```python
from build123d import *

# Parameters (mm, degrees)
F0_W     = 63.5
F0_H     = 15.24
F1_DEPTH = 4.826
F2_W     = 2.667
F2_H     = 5.715
F2_W_2   = 5.715
F2_H_2   = 1.905
F3_DEPTH = 3.175
F4_W     = 63.5
F4_H     = 15.24
F5_DEPTH = 2.54
F7_D     = 7.1374
F8_R     = 5.08


with BuildPart() as f1:
    # F0 (on Top) → F1 (new body)
    with BuildSketch(Plane.XY):
        Rectangle(F0_W, F0_H)
        Polygon((-3.2995567884, -5.715), (-6.5991135768, 0), (-3.2995567884, 5.715), (3.2995567884, 5.715), (6.5991135768, 0), (3.2995567884, -5.715), align=None, mode=Mode.SUBTRACT)
    extrude(amount=F1_DEPTH)

    # F2 (on face) → F3 (join)
    with BuildSketch(Plane.XY.offset(4.826)):
        with Locations((-30.4165, 0)):
            Rectangle(F2_W, F2_H)
        with Locations((-18.1081227605, -6.6675)):
            Rectangle(F2_W_2, F2_H_2)
        with Locations((18.1081227605, -6.6675)):
            Rectangle(F2_W_2, F2_H_2)
        with Locations((-18.1081227605, 6.6675)):
            Rectangle(F2_W_2, F2_H_2)
        with Locations((18.1081227605, 6.6675)):
            Rectangle(F2_W_2, F2_H_2)
        with Locations((30.4165, 0)):
            Rectangle(F2_W, F2_H)
    extrude(amount=F3_DEPTH)

    # F4 (on face) → F5 (join)
    with BuildSketch(Plane(origin=(0, 0, 0), x_dir=(1, 0, 0), z_dir=(0, 0, -1))):
        Rectangle(F4_W, F4_H)
    extrude(amount=F5_DEPTH)

    # F7 (through all)
    with Locations(Plane(origin=(0, 0, -2.54), x_dir=(1, 0, 0), z_dir=(0, 0, -1))):
        with Locations((0, 0)):
            Hole(F7_D / 2)

    # F8
    f8_edges = [f1.edges().sort_by_distance(p)[0] for p in [
        (31.75, -7.62, 1.143),
        (31.75, 7.62, 1.143),
        (-31.75, 7.62, 1.143),
        (-31.75, -7.62, 1.143),
    ]]
    fillet(f8_edges, radius=F8_R)


solid = f1.part
```
The listing builds one solid part. Answer for the finished solid, in the listing's coordinates (mm). A direction names the side the tool comes from. Round coordinates to 2 decimals unless told otherwise and drop trailing zeros. Write each loop counter-clockwise with the first axis right and the second up, starting at its lowest first coordinate (ties: lowest second). Pieces come first, ordered by that corner, then holes. Notation, with made-up numbers: (63, 68.25) -> (67, 68.25) arc R21 cw to (67, 101.25) -> close; hole circle Ø8 at (86, 4.25). An arc over 180 degrees is marked (long way). Answer as a JSON object with one key per item and string values. Group by question number.
Q1. Section C-C (x = 16) is taken. Write down the section's boundary in (y, z) (3 decimals), plus the area to 3 significant figures.
Q2. Straight lines are drawn through the part: line 1 along Y through (x, z) = (0, -1.1); line 2 along Y through (x, z) = (-1.5, 3.5) (3 decimals); line 3 along X through (y, z) = (6, 5). For each, find the intervals that lie inside material, in ascending order.
Q3. Section D-D (x = -23) is taken. Write down the section's boundary in (y, z).
Q4. Section B-B (x = 0) is taken. Write down the section's boundary in (y, z) (3 decimals).
Q5. Section A-A (z = 1) is taken. Write down the section's boundary in (x, y) (3 decimals).
Q6. Determine the mould class of faces 4 (the face through (-4.97, 2.82, 2.38)), 5 (the face through (30.222, -6.171, 1.633)), 6 (the face through (30, -2.858, 6)) for opening direction X: pulls with the +X half, pulls with the -X half, needs draft (parallel to the pull), parting line crosses it, or undercut.
Q7. Which of the six approach directions +Z, -Z, +X, -X, +Y, -Y give full straight-line access (tool end or side, diameter ignored) to faces 1 (the face through (15.251, 7, 6)), 2 (the face through (-30, -2.858, 6)), 3 (the face through (18, 5.715, 6))?
Q8. Each of these flat-tipped pins is pushed along its axis until it touches: pin 1 Ø1.3 at (x, z) = (-30, 6.5) entering from +Y; pin 2 Ø0.6 at (y, z) = (7, 6.5) entering from +X; pin 3 Ø4 at (y, z) = (-6, 3) entering from -X. Where does it stop, or does it pass through?
Check values:
{
 "1": {"outline": "(-7.62, -2.54) -> (7.62, -2.54) -> (7.62, 8.001) -> (5.715, 8.001) -> (5.715, 4.826) -> (-5.715, 4.826) -> (-5.715, 8.001) -> (-7.62, 8.001) -> close", "area": "124 mm^2"},
 "2": {"line 1": "-7.62 to -3.57, 3.57 to 7.62", "line 2": "-7.62 to -5.715, 5.715 to 7.62", "line 3": "-20.97 to -15.25, 15.25 to 20.97"},
 "3": {"outline": "(-7.62, -2.54) -> (7.62, -2.54) -> (7.62, 4.83) -> (-7.62, 4.83) -> close"},
 "4": {"outline": "(-7.62, -2.54) -> (-3.569, -2.54) -> (-3.569, 0) -> (-5.715, 0) -> (-5.715, 4.826) -> (-7.62, 4.826) -> close; (3.569, -2.54) -> (7.62, -2.54) -> (7.62, 4.826) -> (5.715, 4.826) -> (5.715, 0) -> (3.569, 0) -> close"},
 "5": {"outline": "(-31.75, -2.54) arc R5.08 ccw to (-26.67, -7.62) -> (26.67, -7.62) arc R5.08 ccw to (31.75, -2.54) -> (31.75, 2.54) arc R5.08 ccw to (26.67, 7.62) -> (-26.67, 7.62) arc R5.08 ccw to (-31.75, 2.54) -> close; hole (-6.599, 0) -> (-3.3, -5.715) -> (3.3, -5.715) -> (6.599, 0) -> (3.3, 5.715) -> (-3.3, 5.715) -> close"},
 "6": {"face 4": "undercut", "face 5": "pulls with the +X half", "face 6": "needs draft"},
 "7": {"face 1": "+Z, +Y, -Y", "face 2": "+Z, +X, -X, -Y", "face 3": "+Z, +X, -X"},
 "8": {"pin 1": "y = 2.86", "pin 2": "x = 20.97", "pin 3": "x = -31.54"}
}
